Design review of the part built by this model. Coordinates are the model's own, in mm. A direction names the side the tool comes from. Give positions to 0.01 mm unless a question says otherwise; leave off trailing zeros. Order: outer loops, then holes, each group sorted by start corner. A loop starts at its lowest first (then second) coordinate and runs counter-clockwise, first axis right, second up. Notation, with made-up numbers: (66, -14) -> (71, -14) arc R13 ccw to (71, -6) -> close; hole circle Ø11 at (7.5, 18). An arc over 180 degrees is marked (long way). Return JSON: item names as keys, results as strings.
```python
from build123d import *

# Parameters (mm, degrees)
SKETCH003_W     = 3
SKETCH003_H     = 17
POCKET_DEPTH    = 11
SKETCH004_R     = 3.5
POCKET001_DEPTH = 15
SKETCH005_R     = 2
POCKET002_DEPTH = 18
POCKET003_DEPTH = 3.5
PAD_DEPTH       = 4
PAD001_DEPTH    = 1


with BuildPart() as part:
    # Sketch → Revolution (revolve)
    with BuildSketch(Plane.XZ):
        with BuildLine():
            Line((14.4, 0), (14.4, 10.3))
            Line((14.4, 10.3), (19.7, 10.3))
            ThreePointArc((19.7, 10.3), (21.39536, 6.949122), (24.9, 5.6))
            Line((24.9, 1.6), (24.9, 5.6))
            Line((18, 1.6), (24.9, 1.6))
            Line((18, 0), (18, 1.6))
            Line((14.4, 0), (18, 0))
        make_face()
    revolve(axis=Axis((0, 0, 0), (0, 0, 1)))

    # Sketch002 → AdditiveLoft section 0
    with BuildSketch(Plane.XY.offset(5.6)):
        with BuildLine():
            ThreePointArc((-11.510788, -22.079668), (-0.006082, -24.899999), (11.5, -22.085289))
            Line((13.443585, -14.4), (11.5, -22.085289))
            Line((-13.443585, -14.4), (13.443585, -14.4))
            Line((-11.510788, -22.079668), (-13.443585, -14.4))
        make_face()
    # Sketch001 → AdditiveLoft section 1
    with BuildSketch(Plane.XY.offset(10.3)):
        with BuildLine():
            ThreePointArc((-11.510788, -24.423386), (-0.005962, -26.999999), (11.5, -24.428467))
            Line((13.443585, -14.4), (11.5, -24.428467))
            Line((-13.443585, -14.4), (13.443585, -14.4))
            Line((-11.510788, -24.423386), (-13.443585, -14.4))
        make_face()
    loft()

    # Sketch003 → Pocket (cut)
    with BuildSketch(Plane.XY):
        with Locations((0, -20.5)):
            Rectangle(SKETCH003_W, SKETCH003_H)
    extrude(amount=POCKET_DEPTH, mode=Mode.SUBTRACT)

    # Sketch004 → Pocket001 (cut)
    with BuildSketch(Plane.YZ.offset(-22)):
        with Locations((-19.65, 5.95)):
            Circle(SKETCH004_R)
    extrude(amount=POCKET001_DEPTH, mode=Mode.SUBTRACT)

    # Sketch005 → Pocket002 (cut)
    with BuildSketch(Plane.YZ.offset(-7)):
        with Locations((-19.65, 5.95)):
            Circle(SKETCH005_R)
    extrude(amount=POCKET002_DEPTH, mode=Mode.SUBTRACT)

    # Sketch006 → Pocket003 (cut)
    with BuildSketch(Plane.YZ.offset(5.5)):
        Polygon((-16.185898, 3.950001), (-16.185899, 7.950001), (-16.185899, 15.950001), (-23.114102, 15.95), (-23.114102, 3.950001), (-19.65, 1.95), align=None)
    extrude(amount=POCKET003_DEPTH, mode=Mode.SUBTRACT)

    # Sketch007 → Pad (join)
    with BuildSketch(Plane.XY.offset(1.6)):
        with BuildLine():
            ThreePointArc((-14.87057, 19.971884), (-21.967056, 11.724267), (-24.869203, 1.238045))
            Line((-30.912244, 8.027651), (-24.869203, 1.238045))
            Line((-14.87057, 19.971884), (-30.912244, 8.027651))
        make_face()
        with BuildLine():
            Line((14.870569, 19.971885), (30.983027, 8.123311))
            Line((30.983027, 8.123311), (24.87227, 1.174812))
            ThreePointArc((24.87227, 1.174812), (21.981943, 11.696333), (14.870569, 19.971885))
        make_face()
    extrude(amount=PAD_DEPTH)

    # Sketch008 → Pad001 (join)
    with BuildSketch(Plane.XY.offset(0.6)):
        Polygon((25.386727, 12.252334), (30.983027, 8.123311), (27.935703, 4.669279), align=None)
        Polygon((-25.32744, 12.17221), (-30.912244, 8.027651), (-27.855333, 4.582101), align=None)
    extrude(amount=PAD001_DEPTH)


solid = part.part
```
Item 1: Machinability: for faces 5 (the face through (28, 9, 0.6)), 6 (the face through (-26.61, 8.32, 1.09)), 7 (the face through (-7, 17, 1.6)), 8 (the face through (-25, 9, 5.6)), 9 (the face through (25, 9, 5.6)), which of the approach directions +Z, -Z, +X, -X, +Y, -Y give a long, thin tool a straight path to every point of the face, cutting with its end or side? Answer none if there is none.
Result set:
{"face 5": "-Z, +X, +Y, -Y", "face 6": "-Z, -Y", "face 7": "-Z", "face 8": "+Z, -X, +Y", "face 9": "+Z, +X, +Y"}
Item 2: Add section C-C (z = 3.25). Give the boundary of the cut face in (x, y), plus the area to 3 significant figures.
Result set:
{"outline": "(-30.91, 8.03) -> (-24.87, 1.24) arc R24.9 ccw to (-17.79, -17.42) -> (-7, -17.42) -> (-7, -21.88) -> (-11.89, -21.88) arc R24.9 ccw to (-1.5, -24.85) -> (-1.5, -14.32) arc R14.4 cw (long way) to (1.5, -14.32) -> (1.5, -24.85) arc R24.9 ccw to (24.87, 1.17) -> (30.98, 8.12) -> (14.87, 19.97) arc R24.9 ccw to (-14.87, 19.97) -> close; hole (5.5, -21.9) -> (9, -21.9) -> (9, -17.4) -> (5.5, -17.4) -> close", "area": "1,330 mm^2"}
Item 3: Mouldability with a two-part tool opening along Y and no side actions: class faces 1 (the face through (7.226, -21.406, 2.964)), 2 (the face through (-29.405, 6.329, 1.093)), 3 (the face through (-1.5, -21, 4)), 4 (the face through (0.2, 24.9, 3.6)) as released by +Y, released by -Y, zero draft, split by the parting line, or undercut.
Result set:
{"face 1": "undercut", "face 2": "released by -Y", "face 3": "zero draft", "face 4": "released by +Y"}
Item 4: For pin 1 (2 mm diameter, centred on x = 29, y = 9.5, fed in from +Z); pin 2 (5 mm diameter, centred on x = 1.5, z = 4.5, fed in from +Y); pin 3 (4 mm diameter, centred on x = -2.5, z = 5.5, fed in from -Y), all flat-tipped, find the tip position at first contact; note any pin that passes through.
Result set:
{"pin 1": "stops at z = 5.6", "pin 2": "stops at y = 24.9", "pin 3": "stops at y = -25.65"}
Item 5: Wall thickness on L1, parallel to Z at x = -10.5, y = -19.65; L2, parallel to Z at x = 4, y = -19.65; L3, parallel to X at y = -0.5, z = 3: over which ranges is each line inside the solid? List them lowest first. Write a range as [from, to].
Result set:
{"L1": "z = [1.6, 2.45], [9.45, 10.3]", "L2": "z = [1.6, 3.95], [7.95, 10.3]", "L3": "x = [-24.89, -14.39], [14.39, 24.89]"}
Item 6: Add section A-A (y = 0). Give the boundary of the cut face in (x, z).
Result set:
{"outline": "(-24.9, 1.6) -> (-18, 1.6) -> (-18, 0) -> (-14.4, 0) -> (-14.4, 10.3) -> (-19.7, 10.3) arc R5.23 cw to (-24.9, 5.6) -> close; (14.4, 0) -> (18, 0) -> (18, 1.6) -> (24.9, 1.6) -> (24.9, 5.6) arc R5.23 cw to (19.7, 10.3) -> (14.4, 10.3) -> close"}
Item 7: Add section B-B (x = 0). Give the boundary of the cut face in (y, z), plus the area to 3 significant figures.
Result set:
{"outline": "(14.4, 0) -> (18, 0) -> (18, 1.6) -> (24.9, 1.6) -> (24.9, 5.6) arc R5.23 cw to (19.7, 10.3) -> (14.4, 10.3) -> close", "area": "78.4 mm^2"}
